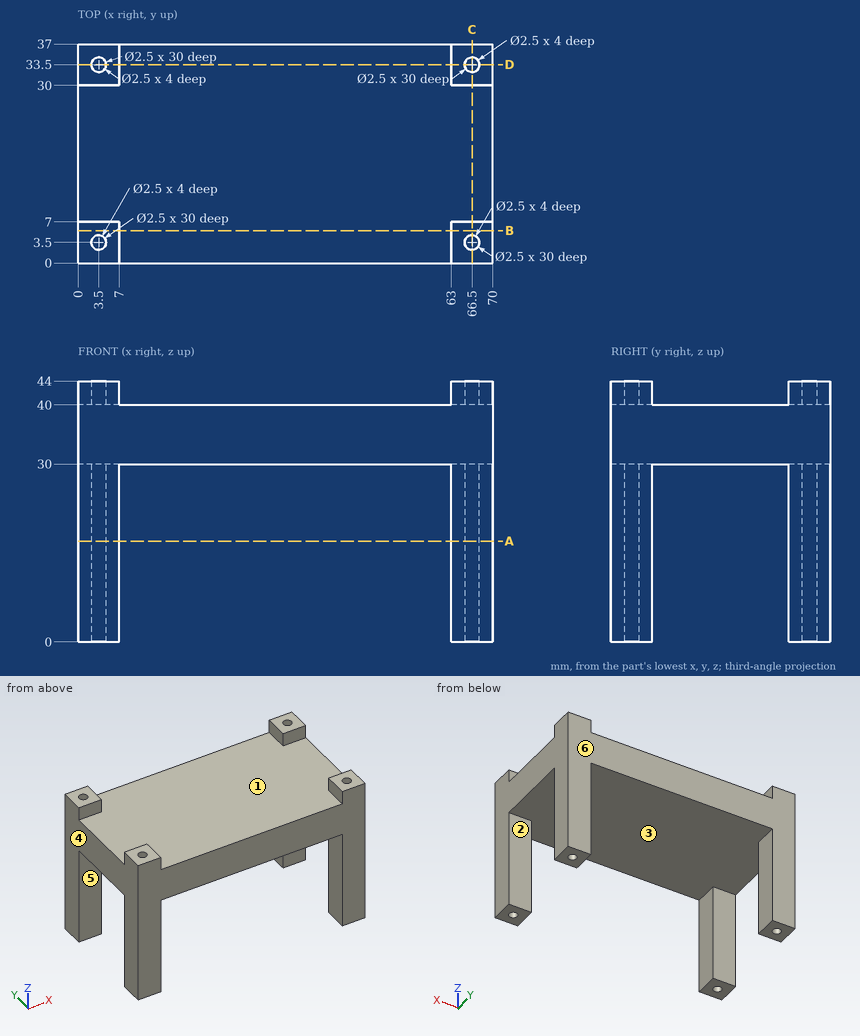
The figure shows three views and two pictorial views of one solid part (mm, origin at its lowest corner). Answer the questions. A direction names the side the tool comes from. Coordinates: 2 decimals unless noted, no trailing zeros. Write each loop counter-clockwise with the first axis right and the second up, starting at its lowest first coordinate (ties: lowest second). Pieces come first, ordered by that corner, then holes. Notation, with made-up numbers: M 41.25,9 L 70.25,9 A23 cw 70.25,28 Z; hole C -2.75,34.5 d10. An arc over 180 degrees is marked long. Answer as CSV lines item,"result". Start each with the question number.
Item 1: Section D-D on y = 33.5 is taken. Write down the section's boundary in (x, z).
Item 2: Section C-C on x = 66.5 is taken. Write down the section's boundary in (y, z).
Item 3: A tool of negligible diameter and unlimited length cuts with its end or side. For the marked faces 1, 2 and 3, from which of +Z, -Z, +X, -X, +Y, -Y can it reach the whole face along a straight path? Write none if from no direction.
Item 4: Flat-ended cylindrical pins translate along their axes: P1, Ø1.5, axis at x = 3.5, y = 3.5, coming from the +Z side; P2, Ø12, axis at x = 26, y = 7.5, coming from the -Z side. Find the tip coordinate at first contact, or state that the pin passes through.
Item 5: Section B-B on y = 5.5 is taken. Write down the section's boundary in (x, z), and give its area (3 significant figures).
Item 6: Determine the mould class of the marked faces 4, 5 and 6 for opening direction Y: released by +Y, released by -Y, zero draft, split by the parting line, or undercut.
Item 7: Section A-A on z = 17 is taken. Write down the section's boundary in (x, y).
Item 8: Consider L1, parallel to Y at x = 3.5, z = 42.55; L2, parallel to X at y = 3.5, z = 20; L3, parallel to X at y = 31, z = 10. Determine where each line is inside the solid, lowest interval first.
Checks:
1,outline,"M 0,0 L 2.25,0 L 2.25,30 L 4.75,30 L 4.75,0 L 7,0 L 7,30 L 63,30 L 63,0 L 65.25,0 L 65.25,30 L 67.75,30 L 67.75,0 L 70,0 L 70,44 L 67.75,44 L 67.75,40 L 65.25,40 L 65.25,44 L 63,44 L 63,40 L 7,40 L 7,44 L 4.75,44 L 4.75,40 L 2.25,40 L 2.25,44 L 0,44 Z"
2,outline,"M 0,0 L 2.25,0 L 2.25,30 L 4.75,30 L 4.75,0 L 7,0 L 7,30 L 30,30 L 30,0 L 32.25,0 L 32.25,30 L 34.75,30 L 34.75,0 L 37,0 L 37,44 L 34.75,44 L 34.75,40 L 32.25,40 L 32.25,44 L 30,44 L 30,40 L 7,40 L 7,44 L 4.75,44 L 4.75,40 L 2.25,40 L 2.25,44 L 0,44 Z"
3,face 1,"+Z"
3,face 2,"-Z, +X, -X"
3,face 3,"-Z"
4,P1,"stops at z = 40"
4,P2,"stops at z = 30"
5,outline,"M 0,0 L 7,0 L 7,30 L 63,30 L 63,0 L 70,0 L 70,44 L 63,44 L 63,40 L 7,40 L 7,44 L 0,44 Z"
5,area,"1,180 mm²"
6,face 4,"zero draft"
6,face 5,"undercut"
6,face 6,"released by +Y"
7,outline,"M 0,0 L 7,0 L 7,7 L 0,7 Z; M 0,30 L 7,30 L 7,37 L 0,37 Z; M 63,0 L 70,0 L 70,7 L 63,7 Z; M 63,30 L 70,30 L 70,37 L 63,37 Z; hole C 3.5,3.5 d2.5; hole C 3.5,33.5 d2.5; hole C 66.5,3.5 d2.5; hole C 66.5,33.5 d2.5"
8,L1,"y = 0 to 2.25, 4.75 to 7, 30 to 32.25, 34.75 to 37"
8,L2,"x = 0 to 2.25, 4.75 to 7, 63 to 65.25, 67.75 to 70"
8,L3,"x = 0 to 7, 63 to 70"
